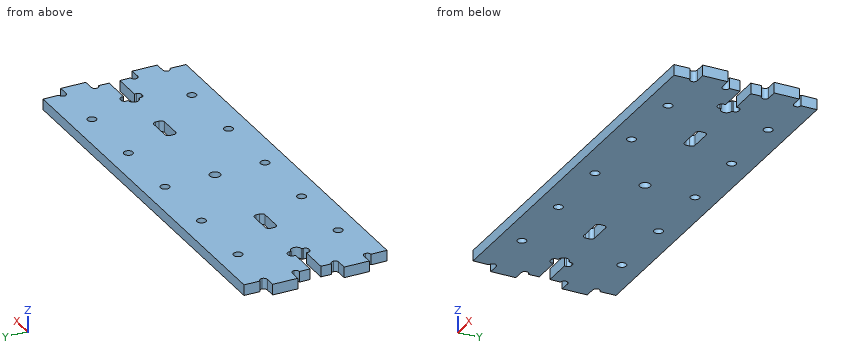
from build123d import *

# Parameters (mm, degrees)
SKETCH1_W           = 110
SKETCH1_H           = 40
BOSS_EXTRUDE1_DEPTH = 3
BOSS_EXTRUDE2_DEPTH = 3
SKETCH3_R           = 1.5
CUT_EXTRUDE1_DEPTH  = 3
SKETCH4_W           = 8
SKETCH4_H           = 3
SKETCH4_W_2         = 2.4
SKETCH4_H_2         = 6
CUT_EXTRUDE2_DEPTH  = 3
FILLET6_R           = 1
SKETCH5_W           = 8
SKETCH5_H           = 3
CUT_EXTRUDE3_DEPTH  = 10
FILLET7_R           = 1
SKETCH6_R           = 1.25
CUT_EXTRUDE4_DEPTH  = 62.424750712


with BuildPart() as part:
    # Sketch1 → Boss-Extrude1 (new body)
    with BuildSketch(Plane.XY):
        Rectangle(SKETCH1_W, SKETCH1_H)
    extrude(amount=BOSS_EXTRUDE1_DEPTH)

    # Sketch2 → Boss-Extrude2 (add)
    with BuildSketch(Plane.XY.offset(3)):
        Polygon((58, 10), (58, 13.5), (55, 13.5), (55, 6.5), (58, 6.5), align=None)
        Polygon((55, -10), (55, -6.5), (58, -6.5), (58, -13.5), (55, -13.5), align=None)
        Polygon((-55, 6.5), (-55, 13.5), (-58, 13.5), (-58, 10), (-58, 6.5), align=None)
        Polygon((-55, -13.5), (-55, -10), (-55, -6.5), (-58, -6.5), (-58, -13.5), align=None)
    extrude(amount=-BOSS_EXTRUDE2_DEPTH)

    # Sketch3 → Cut-Extrude1 (cut)
    with BuildSketch(Plane.XY.offset(3)):
        with BuildLine():
            ThreePointArc((-55, -15.5), (-54.292893219, -15.207106781), (-54, -14.5))
            ThreePointArc((-54, -14.5), (-54.292893219, -13.792893219), (-55, -13.5))
            Line((-55, -13.5), (-55, -15.5))
        make_face()
        with BuildLine():
            Line((-55, -15.5), (-55, -13.5))
            ThreePointArc((-55, -13.5), (-56, -14.5), (-55, -15.5))
        make_face()
        with BuildLine():
            ThreePointArc((-54, -5.5), (-54.292893219, -4.792893219), (-55, -4.5))
            Line((-55, -4.5), (-55, -6.5))
            ThreePointArc((-55, -6.5), (-54.292893219, -6.207106781), (-54, -5.5))
        make_face()
        with BuildLine():
            Line((-55, -6.5), (-55, -4.5))
            ThreePointArc((-55, -4.5), (-56, -5.5), (-55, -6.5))
        make_face()
        with BuildLine():
            ThreePointArc((-55, 4.5), (-54.292893219, 4.792893219), (-54, 5.5))
            ThreePointArc((-54, 5.5), (-54.292893219, 6.207106781), (-55, 6.5))
            Line((-55, 6.5), (-55, 4.5))
        make_face()
        with BuildLine():
            Line((-55, 4.5), (-55, 6.5))
            ThreePointArc((-55, 6.5), (-56, 5.5), (-55, 4.5))
        make_face()
        with BuildLine():
            Line((-55, 15.5), (-55, 13.5))
            ThreePointArc((-55, 13.5), (-54.292893219, 13.792893219), (-54, 14.5))
            ThreePointArc((-54, 14.5), (-54.292893219, 15.207106781), (-55, 15.5))
        make_face()
        with BuildLine():
            ThreePointArc((-55, 15.5), (-56, 14.5), (-55, 13.5))
            Line((-55, 13.5), (-55, 15.5))
        make_face()
        Circle(SKETCH3_R)
        with BuildLine():
            ThreePointArc((56, -5.5), (55.707106781, -4.792893219), (55, -4.5))
            Line((55, -4.5), (55, -6.5))
            ThreePointArc((55, -6.5), (55.707106781, -6.207106781), (56, -5.5))
        make_face()
        with BuildLine():
            Line((55, -6.5), (55, -4.5))
            ThreePointArc((55, -4.5), (54, -5.5), (55, -6.5))
        make_face()
        with BuildLine():
            ThreePointArc((55, -15.5), (55.707106781, -15.207106781), (56, -14.5))
            ThreePointArc((56, -14.5), (55.707106781, -13.792893219), (55, -13.5))
            Line((55, -13.5), (55, -15.5))
        make_face()
        with BuildLine():
            Line((55, -15.5), (55, -13.5))
            ThreePointArc((55, -13.5), (54, -14.5), (55, -15.5))
        make_face()
        with BuildLine():
            ThreePointArc((55, 4.5), (55.707106781, 4.792893219), (56, 5.5))
            ThreePointArc((56, 5.5), (55.707106781, 6.207106781), (55, 6.5))
            Line((55, 6.5), (55, 4.5))
        make_face()
        with BuildLine():
            Line((55, 4.5), (55, 6.5))
            ThreePointArc((55, 6.5), (54, 5.5), (55, 4.5))
        make_face()
        with BuildLine():
            Line((55, 15.5), (55, 13.5))
            ThreePointArc((55, 13.5), (55.707106781, 13.792893219), (56, 14.5))
            ThreePointArc((56, 14.5), (55.707106781, 15.207106781), (55, 15.5))
        make_face()
        with BuildLine():
            ThreePointArc((55, 15.5), (54, 14.5), (55, 13.5))
            Line((55, 13.5), (55, 15.5))
        make_face()
    extrude(amount=-CUT_EXTRUDE1_DEPTH, mode=Mode.SUBTRACT)

    # Sketch4 → Cut-Extrude2 (cut)
    with BuildSketch(Plane.XY.offset(3)):
        with Locations((-51, 0)):
            Rectangle(SKETCH4_W, SKETCH4_H)
        Polygon((-47, 3), (-47, 1.5), (-47, -1.5), (-47, -3), (-44.6, -3), (-44.6, -1.5), (-44.6, 1.5), (-44.6, 3), align=None)
        with BuildLine():
            ThreePointArc((-44.6, -1.5), (-43.1, 0), (-44.6, 1.5))
            Line((-44.6, 1.5), (-44.6, -1.5))
        make_face()
        with Locations((45.8, 0)):
            Rectangle(SKETCH4_W_2, SKETCH4_H_2)
        with BuildLine():
            Line((44.6, -1.5), (44.6, 1.5))
            ThreePointArc((44.6, 1.5), (43.1, 0), (44.6, -1.5))
        make_face()
        with Locations((51, 0)):
            Rectangle(SKETCH4_W, SKETCH4_H)
    extrude(amount=-CUT_EXTRUDE2_DEPTH, mode=Mode.SUBTRACT)

    # Fillet6
    fillet6_edges = [part.edges().sort_by_distance(p)[0] for p in [
        (-47, 3, 1.5),
        (-44.6, 3, 1.5),
        (-44.6, -3, 1.5),
        (-47, -3, 1.5),
        (47, 3, 1.5),
        (47, -3, 1.5),
        (44.6, -3, 1.5),
        (44.6, 3, 1.5),
    ]]
    fillet(fillet6_edges, radius=FILLET6_R)

    # Sketch5 → Cut-Extrude3 (cut)
    with BuildSketch(Plane.XY.offset(3)):
        with Locations((-27.5, 0)):
            Rectangle(SKETCH5_W, SKETCH5_H)
        with Locations((27.5, 0)):
            Rectangle(SKETCH5_W, SKETCH5_H)
    extrude(amount=-CUT_EXTRUDE3_DEPTH, mode=Mode.SUBTRACT)

    # Fillet7
    fillet7_edges = [part.edges().sort_by_distance(p)[0] for p in [
        (-23.5, 1.5, 1.5),
        (-23.5, -1.5, 1.5),
        (-31.5, -1.5, 1.5),
        (-31.5, 1.5, 1.5),
        (31.5, 1.5, 1.5),
        (31.5, -1.5, 1.5),
        (23.5, -1.5, 1.5),
        (23.5, 1.5, 1.5),
    ]]
    fillet(fillet7_edges, radius=FILLET7_R)

    # Sketch6 → Cut-Extrude4 (cut, through all)
    with BuildSketch(Plane.XY.offset(3)):
        with Locations((-40, -14)):
            Circle(SKETCH6_R)
        with Locations((-20, -14)):
            Circle(SKETCH6_R)
        with Locations((0, -14)):
            Circle(SKETCH6_R)
        with Locations((20, -14)):
            Circle(SKETCH6_R)
        with Locations((40, -14)):
            Circle(SKETCH6_R)
        with Locations((40, 14)):
            Circle(SKETCH6_R)
        with Locations((20, 14)):
            Circle(SKETCH6_R)
        with Locations((0, 14)):
            Circle(SKETCH6_R)
        with Locations((-20, 14)):
            Circle(SKETCH6_R)
        with Locations((-40, 14)):
            Circle(SKETCH6_R)
    extrude(amount=-CUT_EXTRUDE4_DEPTH, mode=Mode.SUBTRACT)


solid = part.part
Model file for the job. Use its own axes, mm. Give positions to 0.01 mm unless a question says otherwise; leave off trailing zeros. Loops run counter-clockwise (first coordinate to the right, second up) from the corner with the lowest first, then second, coordinate; pieces in that order, holes last.
1) Saw through at C-C (z = 1.85). Count the separate pieces of the cut face and the enclosed holes in it, plus the area to 3 significant figures.
2) Saw through at B-B (x = 20). Write the cut outline in (y, z), plus the area to 3 significant figures.
3) Saw through at A-A (x = 48.5). Write the cut outline in (y, z), plus the area to 3 significant figures.
4) Flat gauge pins, fed straight in: pin 1 Ø0.5 at (y, z) = (0, 1.5) entering from -X; pin 2 Ø1.5 at (y, z) = (-18, 1.5) entering from +X. Where does each tip first touch, or does it go through?
5) Wall check: line 1 (X direction, y = 2, z = 1.75); line 2 (Y direction, x = 20, z = 1.7); line 3 (Y direction, x = -28.5, z = 2.1). Give the ranges that are in metal, low to high.
Answer block:
1. separate pieces: 1
1. enclosed holes: 13
1. area: 4,290 mm2
2. outline: (-20, 0) - (-15.25, 0) - (-15.25, 3) - (-20, 3) - close; (-12.75, 0) - (12.75, 0) - (12.75, 3) - (-12.75, 3) - close; (15.25, 0) - (20, 0) - (20, 3) - (15.25, 3) - close
2. area: 105 mm2
3. outline: (-20, 0) - (-1.5, 0) - (-1.5, 3) - (-20, 3) - close; (1.5, 0) - (20, 0) - (20, 3) - (1.5, 3) - close
3. area: 111 mm2
4. pin 1: stops at x = -43.12
4. pin 2: stops at x = 55
5. line 1: x = -55 to -47, -44.6 to 44.6, 47 to 55
5. line 2: y = -20 to -15.25, -12.75 to 12.75, 15.25 to 20
5. line 3: y = -20 to -1.5, 1.5 to 20
